```python
from build123d import *

# Parameters (mm, degrees)
F0_W     = 15
F0_H     = 15
F1_DEPTH = 6
F2_R     = 1.5
F3_DEPTH = 15
F4_R     = 1.5
F5_DEPTH = 15
F6_R     = 7.202484
F7_DEPTH = 6


with BuildPart() as f1:
    # F0 (on Top) → F1 (new body)
    with BuildSketch(Plane.XY):
        with Locations((-0.751974, 1.514031)):
            Rectangle(F0_W, F0_H)
    extrude(amount=F1_DEPTH)

    # F2 (on face) → F3 (cut)
    with BuildSketch(Plane.XZ.offset(5.985969)):
        with Locations((-6.251974, 3)):
            Circle(F2_R)
    extrude(amount=-F3_DEPTH, mode=Mode.SUBTRACT)

    # F4 (on face) → F5 (cut)
    with BuildSketch(Plane.XZ.offset(5.985969)):
        with Locations((4.748026, 3)):
            Circle(F4_R)
    extrude(amount=-F5_DEPTH, mode=Mode.SUBTRACT)

    # F6 (on face) → F7 (join)
    with BuildSketch(Plane.XY.offset(6)):
        with Locations((-0.751974, 1.514031)):
            Circle(F6_R)
    extrude(amount=F7_DEPTH)


solid = f1.part
```
Input: part model. Units: mm. Frame: model coordinates. A direction names the side the tool comes from. Coordinates: 2 decimals unless noted, no trailing zeros. Write each loop counter-clockwise with the first axis right and the second up, starting at its lowest first coordinate (ties: lowest second). Pieces come first, ordered by that corner, then holes. Notation, with made-up numbers: (10, 87.25) -> (36, 87.25) arc R17 cw to (36, 106.25) -> close; hole circle Ø11 at (44, 2.25). An arc over 180 degrees is marked (long way). Answer as a JSON object with one key per item and string values.
1. First-contact query: P1, Ø1.5, axis at y = 6, z = 10.5, coming from the +X side. Flat tip, straight axial feed; report the tip coordinate or a pass-through.
Result set:
{"P1": "stops at x = 5.41"}
2. Section A-A on x = 5.5. Return the cut outline in (y, z), then the cut area to 3 significant figures.
Result set:
{"outline": "(-5.99, 0) -> (9.01, 0) -> (9.01, 1.7) -> (-5.99, 1.7) -> close; (-5.99, 4.3) -> (9.01, 4.3) -> (9.01, 6) -> (5.09, 6) -> (5.09, 12) -> (-2.06, 12) -> (-2.06, 6) -> (-5.99, 6) -> close", "area": "94.0 mm2"}
3. Section D-D on x = 0.75. Return the cut outline in (y, z), then the cut area to 3 significant figures.
Result set:
{"outline": "(-5.99, 0) -> (9.01, 0) -> (9.01, 6) -> (8.56, 6) -> (8.56, 12) -> (-5.53, 12) -> (-5.53, 6) -> (-5.99, 6) -> close", "area": "175 mm2"}
4. Access query for faces 4 (the face through (-1, -5.986, 3)), 5 (the face through (-5, -5, 6)). Directions: +Z, -Z, +X, -X, +Y, -Y. A direction counts if a zero-diameter tool reaches every point of the face in a straight line with its end or side. Return the directions, or none.
Result set:
{"face 4": "+Z, -Z, +X, -X, -Y", "face 5": "+Z"}
5. Section C-C on y = -4. Return the cut outline in (x, z), then the cut area to 3 significant figures.
Result set:
{"outline": "(-8.25, 0) -> (6.75, 0) -> (6.75, 6) -> (3.88, 6) -> (3.88, 12) -> (-5.39, 12) -> (-5.39, 6) -> (-8.25, 6) -> close; hole circle Ø3 at (-6.25, 3); hole circle Ø3 at (4.75, 3)", "area": "131 mm2"}
6. Section B-B on z = 3.75. Return the cut outline in (x, y).
Result set:
{"outline": "(-8.25, -5.99) -> (-7.55, -5.99) -> (-7.55, 9.01) -> (-8.25, 9.01) -> close; (-4.95, -5.99) -> (3.45, -5.99) -> (3.45, 9.01) -> (-4.95, 9.01) -> close; (6.05, -5.99) -> (6.75, -5.99) -> (6.75, 9.01) -> (6.05, 9.01) -> close"}
7. Mould query, pull axis X, two halves, no side actions, for faces 1 (the face through (-6.468, -2.869, 8.958)), 2 (the face through (6.134, 1.409, 2.425)), 3 (the face through (-1, 9.014, 3)). Classes: released by +X, released by -X, zero draft, split by the parting line, or undercut.
Result set:
{"face 1": "split by the parting line", "face 2": "undercut", "face 3": "zero draft"}
8. Material intervals for line 1 (X direction, y = -4.25, z = 3.25); line 2 (Z direction, x = -7.25, y = 5.5); line 3 (X direction, y = 6, z = 7), sorted ascending. Write a range as from..to.
Result set:
{"line 1": "x = -8.25..-7.73, -4.77..3.27, 6.23..6.75", "line 2": "z = 0..1.88, 4.12..6", "line 3": "x = -6.39..4.88"}
